The listing builds one solid part. Answer for the finished solid, in the listing's coordinates (mm). Face numbers are marked on the shaded views. A direction names the side the tool comes from. Coordinates: 2 decimals unless noted, no trailing zeros. Write each loop counter-clockwise with the first axis right and the second up, starting at its lowest first coordinate (ties: lowest second). Pieces come first, ordered by that corner, then holes. Notation, with made-up numbers: M 65.25,79 L 114.25,79 A28 ccw 114.25,117 Z; hole C 14,86.25 d2. An arc over 180 degrees is marked long. Answer as CSV lines item,"result". Start each with the question number.
```python
from build123d import *

# Parameters (mm, degrees)
BOSS_EXTRUDE1_DEPTH      = 40.64
BOSS_EXTRUDE1_DEPTH_BACK = 0.254
SKETCH1_R                = 33.7312
SKETCH1_R_2              = 28.3972
SKETCH3_R                = 36.9062
SKETCH3_R_2              = 28.144458554
BOSS_EXTRUDE2_DEPTH      = 2.286
CUT_EXTRUDE4_DEPTH       = 70.866
CUT_EXTRUDE4_DEPTH_BACK  = 4.064
SKETCH5_R                = 3.962523409


with BuildPart() as part:
    # Sketch1 → Boss-Extrude1 (new, two sides: drawn at the far end of the back side and taken through both)
    with BuildSketch(Plane.XY.offset(-BOSS_EXTRUDE1_DEPTH_BACK)):
        Circle(SKETCH1_R)
        Circle(SKETCH1_R_2, mode=Mode.SUBTRACT)
    extrude(amount=BOSS_EXTRUDE1_DEPTH + BOSS_EXTRUDE1_DEPTH_BACK)

    # Sketch3 → Boss-Extrude2 (add)
    with BuildSketch(Plane.XY):
        Circle(SKETCH3_R)
        Circle(SKETCH3_R_2, mode=Mode.SUBTRACT)
    extrude(amount=-BOSS_EXTRUDE2_DEPTH)

    # Sketch5 → Cut-Extrude4 (cut, two sides: drawn at the far end of the back side and taken through both)
    with BuildSketch(Plane.XY.offset(-CUT_EXTRUDE4_DEPTH_BACK)):
        with Locations((0, 28.144458554)):
            Circle(SKETCH5_R)
    extrude(amount=CUT_EXTRUDE4_DEPTH + CUT_EXTRUDE4_DEPTH_BACK, mode=Mode.SUBTRACT)


solid = part.part
```
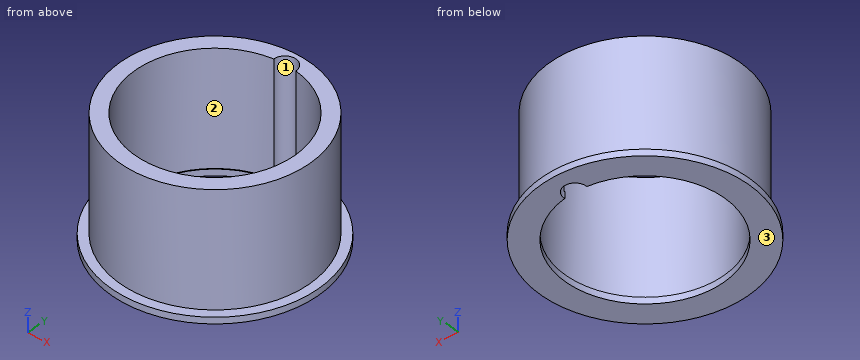
1) The part is cut by section C-C (z = 35.5). Determine the outline of the cut face in (x, y), then the cut area to 3 significant figures.
2) Each of these flat-tipped pins is pushed along its axis until it touches: P1, Ø3, axis at x = 13.5, z = 23, coming from the -Y side; P2, Ø8, axis at x = 19.5, z = 7.5, coming from the -Y side; P3, Ø6, axis at x = 5.5, z = 6, coming from the -Y side. Where does it stop, or does it pass through?
3) Which of the six approach directions +Z, -Z, +X, -X, +Y, -Y give full straight-line access (tool end or side, diameter ignored) to the marked faces 1, 2 and 3?
4) The part is cut by section D-D (x = 31). Determine the outline of the cut face in (y, z).
5) The part is cut by section B-B (x = 0). Determine the outline of the cut face in (y, z).
6) Find the intervals of material crossed by line 1 (X direction, y = 0, z = 13); line 2 (Y direction, x = 0, z = -1); line 3 (Y direction, x = 0, z = 17), in increasing order. Write a range as from..to.
7) The part is cut by section A-A (y = 0). Determine the outline of the cut face in (x, z).
Completed:
1,outline,"C 0,0 d67.46; hole M -3.96,28.12 A28.4 ccw long 3.96,28.12 A3.96 ccw long Z"
1,area,"1,020 mm²"
2,P1,"y = -31.52"
2,P2,"y = -29.96"
2,P3,"y = -33.64"
3,face 1,"+Z, -Z"
3,face 2,"+Z"
3,face 3,"-Z, +X, -X, +Y, -Y"
4,outline,"M -20.03,-2.29 L 20.03,-2.29 L 20.03,0 L 13.3,0 L 13.3,40.64 L -13.3,40.64 L -13.3,0 L -20.03,0 Z"
5,outline,"M -36.91,-2.29 L -28.14,-2.29 L -28.14,0 L -28.4,0 L -28.4,40.64 L -33.73,40.64 L -33.73,0 L -36.91,0 Z; M 32.11,-2.29 L 36.91,-2.29 L 36.91,0 L 33.73,0 L 33.73,40.64 L 32.11,40.64 Z"
6,line 1,"-33.73..-28.4, 28.4..33.73"
6,line 2,"-36.91..-28.14, 32.11..36.91"
6,line 3,"-33.73..-28.4, 32.11..33.73"
7,outline,"M -36.91,-2.29 L -28.14,-2.29 L -28.14,0 L -28.4,0 L -28.4,40.64 L -33.73,40.64 L -33.73,0 L -36.91,0 Z; M 28.14,-2.29 L 36.91,-2.29 L 36.91,0 L 33.73,0 L 33.73,40.64 L 28.4,40.64 L 28.4,0 L 28.14,0 Z"
